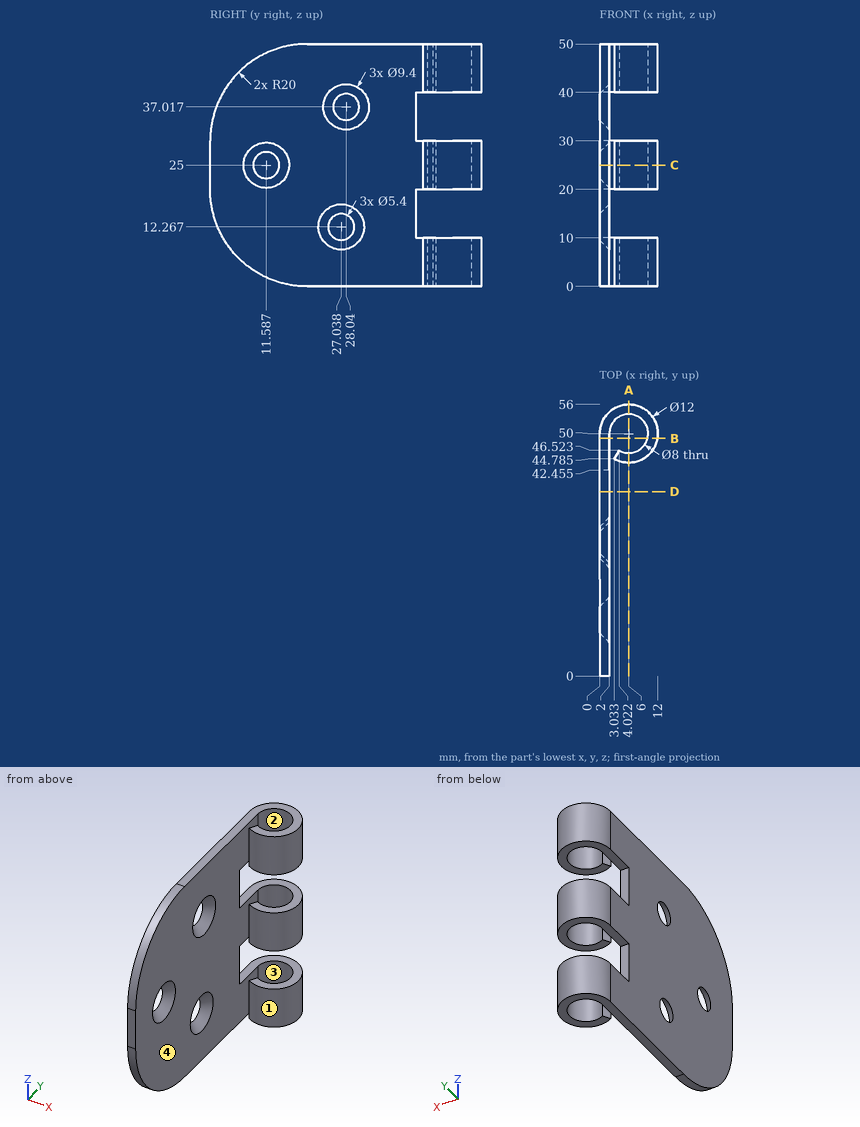
Design review of the part shown in the three views and the two pictorial views. Dimensions are in mm from the part's minimum x, y and z. Round coordinates to 2 decimals unless told otherwise and drop trailing zeros. Loops run counter-clockwise (first coordinate to the right, second up) from the corner with the lowest first, then second, coordinate; pieces in that order, holes last. Notation, with made-up numbers: (38, -14.5) - (48, -14.5) arc R18 ccw to (48, 10.5) - close; hole circle Ø6 at (79, 54.25). An arc over 180 degrees is marked (long way). Write each question's results on one line, items separated by ' | '. Start each with the question number.
Q1. Wall thickness on line 1 along Y through (x, z) = (6, 7.5); line 2 along X through (y, z) = (50, 7); line 3 along X through (y, z) = (34, 34.5): over which ranges is each line inside the solid? List them lowest first. Write a range as [from, to].
Q2. Take a section at C-C on z = 25. Give the boundary of the cut face in (x, y) (1 decimal).
Q3. Take a section at D-D on y = 38. Give the boundary of the cut face in (x, z), plus the area to 3 significant figures.
Q4. Take a section at B-B on y = 49. Give the boundary of the cut face in (x, z), plus the area to 3 significant figures.
Q5. Take a section at A-A on x = 6. Give the boundary of the cut face in (y, z), plus the area to 3 significant figures.
Q6. Insertion check: P1, Ø6, axis at x = 1.5, z = 8, coming from the +Y side; P2, Ø1, axis at x = 1.5, z = 34.5, coming from the +Y side (1 decimal); P3, Ø2, axis at x = 1, y = 10.5, coming from the -Z side (1 decimal); P4, Ø6.5, axis at x = 6, y = 50, coming from the -Z side. Each pin has a flat end and moves straight along its axis. Give the tip position at first contact, or say it passes through.
Q7. Draft analysis for pull direction Y (two halves, no side actions). For the marked faces 1, 2, 3 and 4, state which applies: pulls with the +Y half, pulls with the -Y half, needs draft (parallel to the pull), parting line crosses it, or undercut.
Data:
1) line 1: y = [44, 46], [54, 56] | line 2: x = [0, 2], [10, 12] | line 3: x = [0, 2]
2) outline: (0, 0) - (2, 0) - (2, 6.9) - (0, 8.9) - close; (0, 14.3) - (2, 16.3) - (2, 50) arc R4 cw (long way) to (4, 46.5) - (3, 44.8) arc R6 ccw (long way) to (0, 50) - close
3) outline: (0, 0) - (2, 0) - (2, 50) - (0, 50) - close | area: 100 mm²
4) outline: (0, 0) - (2, 0) - (2, 10) - (0, 10) - close; (0, 20) - (2, 20) - (2, 30) - (0, 30) - close; (0, 40) - (2, 40) - (2, 50) - (0, 50) - close; (9.87, 0) - (11.92, 0) - (11.92, 10) - (9.87, 10) - close; (9.87, 20) - (11.92, 20) - (11.92, 30) - (9.87, 30) - close; (9.87, 40) - (11.92, 40) - (11.92, 50) - (9.87, 50) - close | area: 121 mm²
5) outline: (44, 0) - (46, 0) - (46, 10) - (44, 10) - close; (44, 20) - (46, 20) - (46, 30) - (44, 30) - close; (44, 40) - (46, 40) - (46, 50) - (44, 50) - close; (54, 0) - (56, 0) - (56, 10) - (54, 10) - close; (54, 20) - (56, 20) - (56, 30) - (54, 30) - close; (54, 40) - (56, 40) - (56, 50) - (54, 50) - close | area: 120 mm²
6) P1: stops at y = 55.81 | P2: stops at y = 42.5 | P3: stops at z = 1.9 | P4: passes through
7) face 1: parting line crosses it | face 2: undercut | face 3: undercut | face 4: needs draft
